Verification items for the finished model (mm, model axes). Round coordinates to 2 decimals unless told otherwise and drop trailing zeros. Loops run counter-clockwise (first coordinate to the right, second up) from the corner with the lowest first, then second, coordinate; pieces in that order, holes last. Notation, with made-up numbers: M -38,4 L -31,4 A7 ccw -31,11 Z; hole C -38,-18 d11. An arc over 180 degrees is marked long. Answer as CSV lines item,"result".
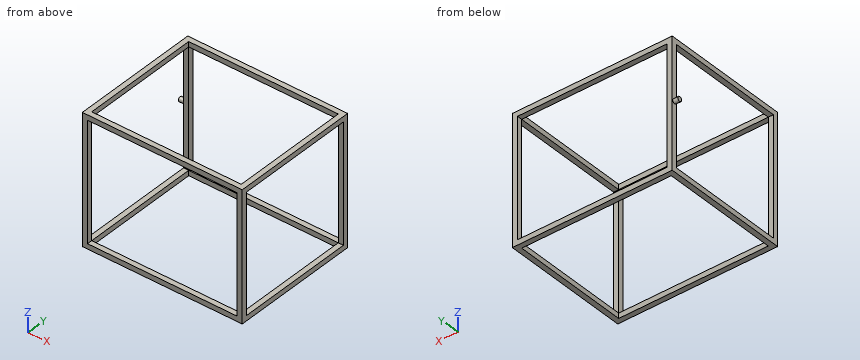
```python
from build123d import *

# Parameters (mm, degrees)
SKETCH_1_W      = 20
SKETCH_1_H      = 20
EXTRUDE_1_DEPTH = 500
SKETCH_2_W      = 20
SKETCH_2_H      = 20
EXTRUDE_2_DEPTH = 580
SKETCH_3_W      = 500
SKETCH_3_H      = 20
EXTRUDE_3_DEPTH = 20
SKETCH_4_W      = 20
SKETCH_4_H      = 20
EXTRUDE_4_DEPTH = 460
SKETCH_5_W      = 620
SKETCH_5_H      = 500
SKETCH_5_W_2    = 580
SKETCH_5_H_2    = 460
EXTRUDE_5_DEPTH = 20
SKETCH_6_R      = 8.86405517
EXTRUDE_6_DEPTH = 20


with BuildPart() as part:
    # 草图1 → 凸台-拉伸1 (new body)
    with BuildSketch(Plane.XY):
        with Locations((10, -10)):
            Rectangle(SKETCH_1_W, SKETCH_1_H)
    extrude(amount=EXTRUDE_1_DEPTH)

    # 草图2 → 凸台-拉伸2 (add)
    with BuildSketch(Plane.ZY):
        with Locations((490, -10)):
            Rectangle(SKETCH_2_W, SKETCH_2_H)
        with Locations((10, -10)):
            Rectangle(SKETCH_2_W, SKETCH_2_H)
    extrude(amount=EXTRUDE_2_DEPTH)

    # 草图3 → 凸台-拉伸3 (add)
    with BuildSketch(Plane.ZY.offset(580)):
        with Locations((250, -10)):
            Rectangle(SKETCH_3_W, SKETCH_3_H)
    extrude(amount=EXTRUDE_3_DEPTH)

    # 草图4 → 凸台-拉伸4 (add)
    with BuildSketch(Plane(origin=(0, 0, 0), x_dir=(1, 0, 0), z_dir=(0, 1, 0))):
        with Locations((10, -10)):
            Rectangle(SKETCH_4_W, SKETCH_4_H)
        with Locations((10, -490)):
            Rectangle(SKETCH_4_W, SKETCH_4_H)
        with Locations((-590, -490)):
            Rectangle(SKETCH_4_W, SKETCH_4_H)
        with Locations((-590, -10)):
            Rectangle(SKETCH_4_W, SKETCH_4_H)
    extrude(amount=EXTRUDE_4_DEPTH)

    # 草图5 → 凸台-拉伸5 (add)
    with BuildSketch(Plane(origin=(0, 460, 0), x_dir=(1, 0, 0), z_dir=(0, 1, 0))):
        with Locations((-290, -250)):
            Rectangle(SKETCH_5_W, SKETCH_5_H)
        with Locations((-290, -250)):
            Rectangle(SKETCH_5_W_2, SKETCH_5_H_2, mode=Mode.SUBTRACT)
    extrude(amount=EXTRUDE_5_DEPTH)

    # 草图6 → 凸台-拉伸6 (add)
    with BuildSketch(Plane.ZY.offset(600)):
        with Locations(Location((262.359920907, 468.86405517, 0), (0, 0, 270))):
            Circle(SKETCH_6_R)
    extrude(amount=EXTRUDE_6_DEPTH)


solid = part.part
```
1) Section check B-B (z = 416). Record the cut outline in (x, y).
Here are the results:
outline,"M -600,-20 L -580,-20 L -580,0 L -600,0 Z; M -600,460 L -580,460 L -580,480 L -600,480 Z; M 0,-20 L 20,-20 L 20,0 L 0,0 Z; M 0,460 L 20,460 L 20,480 L 0,480 Z"
2) Section check A-A (x = -423). Record the cut outline in (y, z), plus the area to 3 significant figures.
Here are the results:
outline,"M -20,0 L 0,0 L 0,20 L -20,20 Z; M -20,480 L 0,480 L 0,500 L -20,500 Z; M 460,0 L 480,0 L 480,20 L 460,20 Z; M 460,480 L 480,480 L 480,500 L 460,500 Z"
area,"1,600 mm^2"
3) Go/stop test with flat-tipped pins: pin 1 (6 mm diameter, centred on x = -377, y = 469.5, fed in from -Z); pin 2 (22 mm diameter, centred on y = -5, z = 358.5, fed in from -X). Record where each tip stops, or that it passes through.
Here are the results:
pin 1,"stops at z = 0"
pin 2,"stops at x = -600"
